```python
from build123d import *

# Parameters (mm, degrees)
SKETCH2_W           = 259.71
SKETCH2_H           = 215.9
BOSS_EXTRUDE1_DEPTH = 5
SKETCH1_R           = 1.75
BOSS_EXTRUDE2_DEPTH = 30
FANS_W              = 27.900833557
FANS_H              = 27.900833558
FANS_W_2            = 38.326934518
FANS_H_2            = 41.851250335
FANS_H_3            = 27.900833557
BOSS_EXTRUDE3_DEPTH = 30


with BuildPart() as part:
    # Sketch2 → Boss-Extrude1 (new body)
    with BuildSketch(Plane(origin=(0, 0, 0), x_dir=(1, 0, 0), z_dir=(0, 1, 0))):
        with Locations((-196.717193813, 0.240534117)):
            Rectangle(SKETCH2_W, SKETCH2_H)
    extrude(amount=BOSS_EXTRUDE1_DEPTH)

    # Sketch1 → Boss-Extrude2 (add)
    with BuildSketch(Plane(origin=(0, 0, 0), x_dir=(1, 0, 0), z_dir=(0, 1, 0))):
        with Locations((-320.092193813, 101.170534117)):
            Circle(SKETCH1_R)
        with Locations((-312.852193813, 99.850534117)):
            Circle(SKETCH1_R)
        with Locations((-318.832193813, -92.309465883)):
            Circle(SKETCH1_R)
        with Locations((-320.102193813, -99.489465883)):
            Circle(SKETCH1_R)
        with Locations((-177.862193813, -34.399465883)):
            Circle(SKETCH1_R)
        with Locations((-170.242193813, -34.399465883)):
            Circle(SKETCH1_R)
        with Locations((-104.382193813, -25.149465883)):
            Circle(SKETCH1_R)
        with Locations((-216.142193813, -6.769465883)):
            Circle(SKETCH1_R)
        with Locations((-77.992193813, -11.859465883)):
            Circle(SKETCH1_R)
        with Locations((-80.702193813, -2.389465883)):
            Circle(SKETCH1_R)
        with Locations((-84.902193813, -98.529465883)):
            Circle(SKETCH1_R)
        with Locations((-79.259756914, -99.489465883)):
            Circle(SKETCH1_R)
        with Locations((-104.372193813, 71.880534117)):
            Circle(SKETCH1_R)
        with Locations((-80.542193813, 80.410534117)):
            Circle(SKETCH1_R)
        with Locations((-75.622193813, 101.170534117)):
            Circle(SKETCH1_R)
        with Locations((-224.842193813, 89.780534117)):
            Circle(SKETCH1_R)
    extrude(amount=-BOSS_EXTRUDE2_DEPTH)

    # fans → Boss-Extrude3 (add)
    with BuildSketch(Plane(origin=(0, 5, 0), x_dir=(1, 0, 0), z_dir=(0, 1, 0))):
        with Locations((-146.055153933, -7.909446212)):
            Rectangle(FANS_W, FANS_H)
        with Locations((-124.395296303, 37.09900371)):
            Rectangle(FANS_W_2, FANS_H_2)
        with Locations((-181.151465618, -8.056292705)):
            Rectangle(FANS_W, FANS_H_3)
        with Locations((-148.478121058, 78.803407554)):
            Rectangle(FANS_W, FANS_H_3)
        with Locations((-183.574432743, 78.656561061)):
            Rectangle(FANS_W, FANS_H_3)
    extrude(amount=BOSS_EXTRUDE3_DEPTH)


solid = part.part
```
Can you work these out from the model? Positions are in its coordinate system, mm. A direction names the side the tool comes from. Coordinates: 2 decimals unless noted, no trailing zeros. Write each loop counter-clockwise with the first axis right and the second up, starting at its lowest first coordinate (ties: lowest second). Pieces come first, ordered by that corner, then holes. Notation, with made-up numbers: M 66.5,15 L 122.5,15 A23 cw 122.5,31 Z; hole C 60,2 d6. An arc over 180 degrees is marked long. Write item = value, one per line. Start each with the question number.
Q1. If we section it at D-D, the plane y = -24.5: State how many separate pieces and enclosed holes the cut face has, then the cut area to 3 significant figures.
Q2. Thinking about a two-plate mould opening in Z: for faces 1 (the face through (-134.528, 20, -79)), 2 (the face through (-143.559, 20, -37)), 3 (the face through (-146, 20, 21.86)), which applies, released by +Z, released by -Z, zero draft, split by the parting line, or undercut?
Q3. On a 3-axis mill with a long thin cutter (end or side, diameter ignored), from which of +Z, -Z, +X, -X, +Y, -Y can I reach the whole of each face in a straight line? I mean faces 4 (the face through (-132.105, 20, 8)), 5 (the face through (-146, 20, -6.041)), 6 (the face through (-169.624, 20, -78)), 7 (the face through (-105.232, 20, -37)), 8 (the face through (-195.102, 20, 8)). Say none if no direction works.
Q4. If we section it at C-C, the plane z = -43: Write out the boundary of the cut face in (x, y).
Q5. If I drill on L1, parallel to X at y = 31, z = -4.5; L2, parallel to Y at x = -258.5, z = 44; L3, parallel to Y at x = -168, z = 0, over which ranges is the centre line in solid material (lowest first)? Write a range as [from, to].
Q6. If we section it at A-A, the plane x = -125: Write out the boundary of the cut face in (y, z), then the cut area to 3 significant figures.
Q7. I'm going to push flat-ended pins straight in: pin 1 (6 mm diameter, centred on x = -96.5, z = 27, fed in from +Y); pin 2 (14 mm diameter, centred on x = -139.5, y = 25.5, fed in from -Z); pin 3 (8.5 mm diameter, centred on y = 24.5, z = 7, fed in from +X). Where does each tip first touch, or does it pass through?
Q8. If we section it at B-B, the plane y = 15: Write out the boundary of the cut face in (x, z), then the cut area to 3 significant figures.
Check sheet entries:
q1.separate_pieces = 16
q1.enclosed_holes = 0
q1.area = 154 mm²
q2.face_1 = zero draft
q2.face_2 = undercut
q2.face_3 = released by +Z
q3.face_4 = +Z, +X, +Y
q3.face_5 = +X, -X, +Y
q3.face_6 = -Z, +Y
q3.face_7 = +Z, -Z, +X, +Y
q3.face_8 = +Z, -X, +Y
q4.outline = M -326.57,0 L -66.86,0 L -66.86,5 L -105.23,5 L -105.23,35 L -143.56,35 L -143.56,5 L -326.57,5 Z
q5.L1 = [-195.1, -167.2], [-160.01, -132.1]
q5.L2 = [0, 5]
q5.L3 = [0, 35]
q6.outline = M 0,-108.19 L 5,-108.19 L 5,-58.02 L 35,-58.02 L 35,-16.17 L 5,-16.17 L 5,107.71 L 0,107.71 Z
q6.area = 2,340 mm²
q7.pin_1 = 5
q7.pin_2 = -92.75
q7.pin_3 = -132.1
q8.outline = M -197.52,-92.61 L -169.62,-92.61 L -169.62,-64.71 L -197.52,-64.71 Z; M -195.1,-5.89 L -167.2,-5.89 L -167.2,22.01 L -195.1,22.01 Z; M -162.43,-92.75 L -134.53,-92.75 L -134.53,-64.85 L -162.43,-64.85 Z; M -160.01,-6.04 L -132.1,-6.04 L -132.1,21.86 L -160.01,21.86 Z; M -143.56,-58.02 L -105.23,-58.02 L -105.23,-16.17 L -143.56,-16.17 Z
q8.area = 4,720 mm²
